```python
from build123d import *

# Parameters (mm, degrees)
SKETCH1_W                                       = 278
SKETCH1_H                                       = 278
BOSS_EXTRUDE1_DEPTH                             = 6.35
CHAMFER1_SIZE                                   = 20
SKETCH4_R                                       = 2.75
CUT_EXTRUDE2_DEPTH                              = 76.2
SKETCH8_R                                       = 16
CUT_EXTRUDE4_DEPTH                              = 105
CSK_FOR_M4_FLAT_HEAD_MACHINE_SCREW2_D           = 4.5
CSK_FOR_M4_FLAT_HEAD_MACHINE_SCREW2_CSINK_D     = 9.4
CSK_FOR_M4_FLAT_HEAD_MACHINE_SCREW2_CSINK_ANGLE = 90
CSK_FOR_M3_FLAT_HEAD_MACHINE_SCREW1_D           = 3.4
CSK_FOR_M3_FLAT_HEAD_MACHINE_SCREW1_CSINK_D     = 6.3
CSK_FOR_M3_FLAT_HEAD_MACHINE_SCREW1_CSINK_ANGLE = 90
CSK_FOR_M3_FLAT_HEAD_MACHINE_SCREW2_D           = 3.4
CSK_FOR_M3_FLAT_HEAD_MACHINE_SCREW2_CSINK_D     = 6.3
CSK_FOR_M3_FLAT_HEAD_MACHINE_SCREW2_CSINK_ANGLE = 90


with BuildPart() as part:
    # Sketch1 → Boss-Extrude1 (new body)
    with BuildSketch(Plane.XY):
        Rectangle(SKETCH1_W, SKETCH1_H)
    extrude(amount=BOSS_EXTRUDE1_DEPTH)

    # Chamfer1
    chamfer1_edges = [part.edges().sort_by_distance(p)[0] for p in [
        (-139, 139, 3.175),
        (139, 139, 3.175),
        (139, -139, 3.175),
        (-139, -139, 3.175),
    ]]
    chamfer(chamfer1_edges, length=CHAMFER1_SIZE)

    # Sketch4 → Cut-Extrude2 (cut)
    with BuildSketch(Plane.XY.offset(6.35)):
        with Locations((-90, 130)):
            Circle(SKETCH4_R)
        with Locations((0, 130)):
            Circle(SKETCH4_R)
        with Locations((90, 130)):
            Circle(SKETCH4_R)
        with Locations((90, -130)):
            Circle(SKETCH4_R)
        with Locations((0, -130)):
            Circle(SKETCH4_R)
        with Locations((-90, -130)):
            Circle(SKETCH4_R)
    extrude(amount=-CUT_EXTRUDE2_DEPTH, mode=Mode.SUBTRACT)

    # Sketch8 → Cut-Extrude4 (cut)
    with BuildSketch(Plane.XY.offset(6.35)):
        with Locations((0, 89)):
            Circle(SKETCH8_R)
        with Locations((0, -89)):
            Circle(SKETCH8_R)
    extrude(amount=-CUT_EXTRUDE4_DEPTH, mode=Mode.SUBTRACT)

    # CSK for M4 Flat Head Machine Screw2 (through all)
    with Locations(Plane.XY.offset(6.35)):
        with Locations((-27.5, 89), (27.5, 89), (27.5, -89), (-27.5, -89)):
            CounterSinkHole(CSK_FOR_M4_FLAT_HEAD_MACHINE_SCREW2_D / 2, CSK_FOR_M4_FLAT_HEAD_MACHINE_SCREW2_CSINK_D / 2, counter_sink_angle=CSK_FOR_M4_FLAT_HEAD_MACHINE_SCREW2_CSINK_ANGLE)

    # CSK for M3 Flat Head Machine Screw1 (through all)
    with Locations(Plane.XY.offset(6.35)):
        with Locations((-131, 30), (-120, 30), (-120, -30), (-131, -30), (131, -30), (120, -30), (120, 30), (131, 30)):
            CounterSinkHole(CSK_FOR_M3_FLAT_HEAD_MACHINE_SCREW1_D / 2, CSK_FOR_M3_FLAT_HEAD_MACHINE_SCREW1_CSINK_D / 2, counter_sink_angle=CSK_FOR_M3_FLAT_HEAD_MACHINE_SCREW1_CSINK_ANGLE)

    # CSK for M3 Flat Head Machine Screw2 (through all)
    with Locations(Plane.XY.offset(6.35)):
        with Locations((-47.23657748, -43.137455791), (-51.23657748, 39.362544209), (28.26342252, 51.862544209), (28.26342252, -51.137455791)):
            CounterSinkHole(CSK_FOR_M3_FLAT_HEAD_MACHINE_SCREW2_D / 2, CSK_FOR_M3_FLAT_HEAD_MACHINE_SCREW2_CSINK_D / 2, counter_sink_angle=CSK_FOR_M3_FLAT_HEAD_MACHINE_SCREW2_CSINK_ANGLE)


solid = part.part
```
Build history of the part. All positions in model axes, mm. Coordinates: 2 decimals unless noted, no trailing zeros.
1. Pull direction X, two halves, no side cores. Call faces 1 (the flat face through (-129, 129, 3)), 2 (the flat face through (-2, -139, 3)), 3 (the conical face through (-27.19, 91.35, 4.02)): released by +X, released by -X, zero draft, split by the parting line, or undercut.
Answer block:
face 1: released by -X
face 2: zero draft
face 3: undercut
2. Drop flat-ended pins along their axis: pin 1 (5 mm diameter, centred on x = 0, y = 130, fed in from +Z); pin 2 (5 mm diameter, centred on x = -27.5, y = -89, fed in from +Z); pin 3 (6.5 mm diameter, centred on x = 0, y = -130, fed in from -Z); pin 4 (7 mm diameter, centred on x = 27.5, y = 89, fed in from +Z). Give the stop position or say it passes through.
Answer block:
pin 1: passes through
pin 2: stops at z = 4.15
pin 3: stops at z = 0
pin 4: stops at z = 5.15
3. Drill centre lines: probe 1 along X at (y, z) = (30, 1.9); probe 2 along Y at (x, z) = (-90, 2.25); probe 3 along Y at (x, z) = (-27.5, 0.9). Where is each one in solid material? Low to high.
Answer block:
probe 1: x = -139 to -132.7, -129.3 to -121.7, -118.3 to 118.3, 121.7 to 129.3, 132.7 to 139
probe 2: y = -139 to -132.75, -127.25 to 127.25, 132.75 to 139
probe 3: y = -139 to -91.25, -86.75 to 86.75, 91.25 to 139
